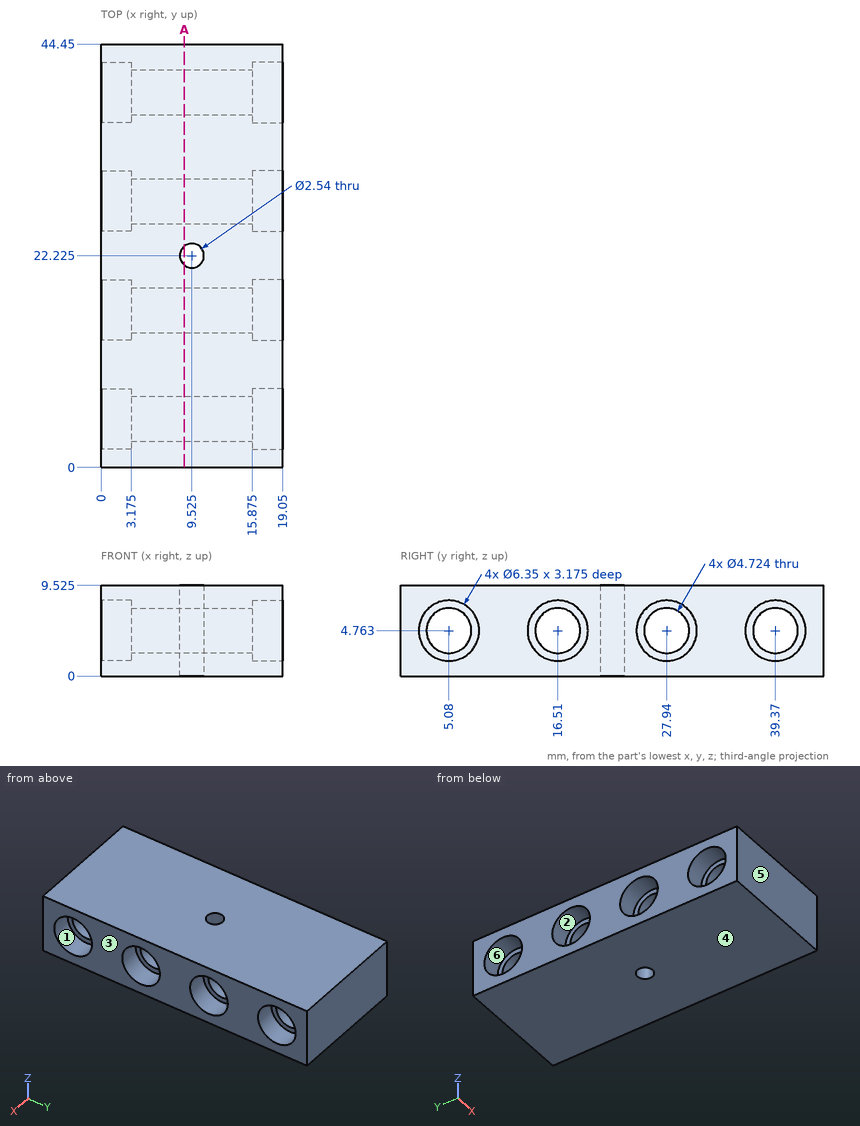
Source: three-view drawing plus pictorial views. Frame: mm from the lowest corner of the part. A direction names the side the tool comes from. Coordinates: 2 decimals unless noted, no trailing zeros. Write each question's results on one line, items separated by ' | '. Start each with the question number.
1. Pin query (flat end, axial travel): pin 1 (5 mm diameter, centred on x = 11, z = 7.5, fed in from -Y); pin 2 (3 mm diameter, centred on y = 5.5, z = 6, fed in from -X) (1 decimal); pin 3 (5.5 mm diameter, centred on y = 39.37, z = 4.76, fed in from +X) (1 decimal). Return the tip coordinate at first contact, or that it passes through.
2. Draft query along Z for the marked faces 4, 5 and 6. Return one class per face: +Z half, -Z half, draft (parallel to the pull), parting line (faces both ways), or undercut.
3. Reachability of the marked faces 1, 2 and 3 from +Z, -Z, +X, -X, +Y, -Y: full face, straight path, thin tool, end or side. Return the list, or none.
4. Material intervals for L1, parallel to Z at x = 1.6, y = 5.08 (1 decimal); L2, parallel to Y at x = 13, z = 4.5; L3, parallel to X at y = 14, z = 5 (1 decimal), sorted ascending.
5. Section A-A, the plane x = 8.75. State how many separate pieces and enclosed holes the cut face has, then the cut area to 3 significant figures.
Solution:
1) pin 1: y = 0 | pin 2: x = 3.2 | pin 3: x = 15.9
2) face 4: -Z half | face 5: draft | face 6: undercut
3) face 1: +X | face 2: -X | face 3: +Z, -Z, +X, +Y, -Y
4) L1: 0 to 1.6, 7.9 to 9.5 | L2: 0 to 2.73, 7.43 to 14.16, 18.86 to 25.59, 30.29 to 37.02, 41.72 to 44.45 | L3: 3.2 to 15.9
5) separate pieces: 2 | enclosed holes: 4 | area: 334 mm²
